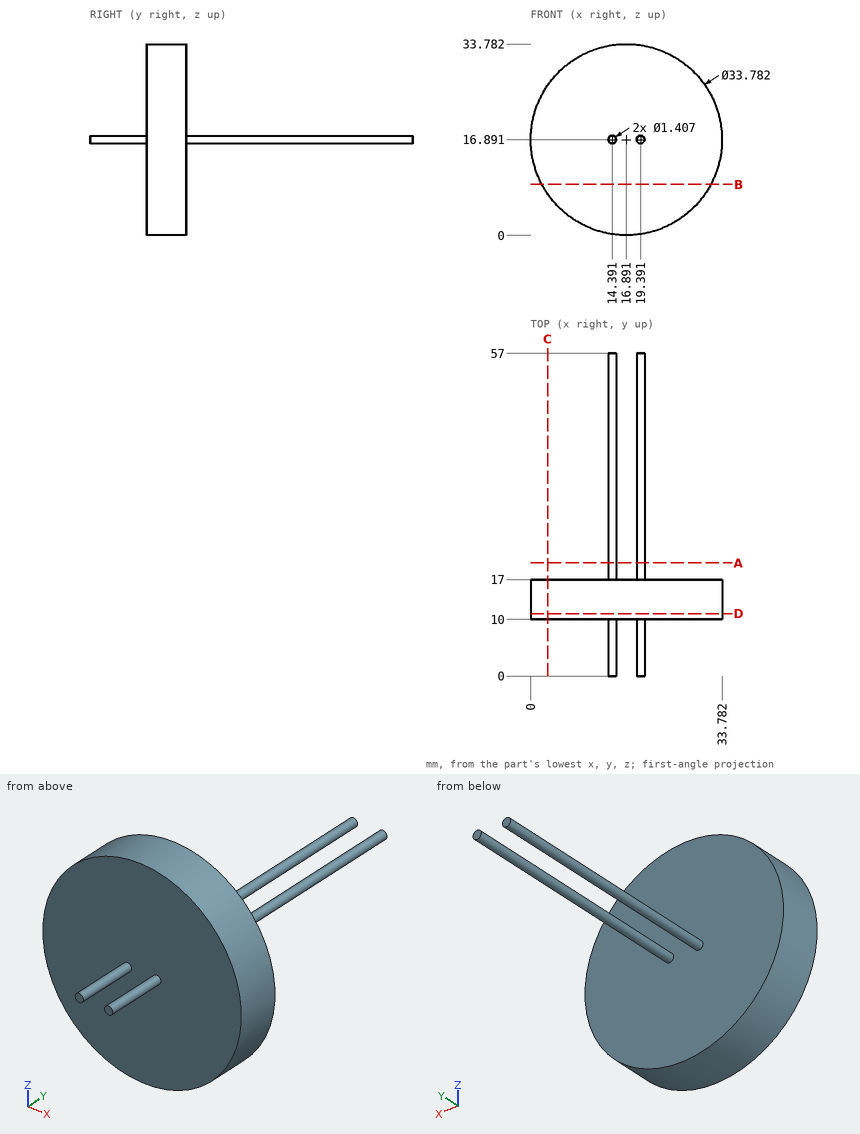
Design review of the part shown in the three views and the two pictorial views. Dimensions are in mm from the part's minimum x, y and z. Round coordinates to 2 decimals unless told otherwise and drop trailing zeros. Write each loop counter-clockwise with the first axis right and the second up, starting at its lowest first coordinate (ties: lowest second). Pieces come first, ordered by that corner, then holes. Notation, with made-up numbers: (-9, 58.5) - (18, 58.5) arc R26 cw to (18, 93.5) - close; hole circle Ø10 at (78, -1). An arc over 180 degrees is marked (long way). Write item = value, one per line. Start each with the question number.
1. Consider section C-C on x = 3. State the section outline as (y, z) points, plus the area to 3 significant figures.
2. Wall thickness on L1, parallel to Y at x = 12, z = 23.5; L2, parallel to Z at x = 30, y = 16.5; L3, parallel to X at y = 12, z = 4.5: over which ranges is each line inside the solid? List them lowest first.
3. Consider section B-B on z = 9. State the section outline as (x, y) points (1 decimal), plus the area to 3 significant figures.
4. Consider section A-A on y = 20. State the section outline as (x, z) points (1 decimal).
5. For pin 1 Ø10 at (x, y) = (29.5, 20.5) entering from -Z; pin 2 Ø10 at (x, z) = (4, 21) entering from +Y; pin 3 Ø4 at (y, z) = (23, 16) entering from +X, all flat-tipped, find the tip position at first contact; note any pin that passes through.
6. Consider section D-D on y = 11. State the section outline as (x, z) points.
Evaluation:
q1.outline = (10, 7.28) - (17, 7.28) - (17, 26.5) - (10, 26.5) - close
q1.area = 135 mm2
q2.L1 = 10 to 17
q2.L2 = 6.24 to 27.54
q2.L3 = 5.41 to 28.37
q3.outline = (2, 10) - (31.8, 10) - (31.8, 17) - (2, 17) - close
q3.area = 209 mm2
q4.outline = circle Ø1.4 at (14.4, 16.9); circle Ø1.4 at (19.4, 16.9)
q5.pin_1 = 2.62
q5.pin_2 = 17
q5.pin_3 = 20.09
q6.outline = circle Ø33.78 at (16.89, 16.89)
